The model under review builds one solid part; all positions refer to its coordinate system, in mm. Face numbers are marked on the shaded views. A direction names the side the tool comes from. Round coordinates to 2 decimals unless told otherwise and drop trailing zeros. Loops run counter-clockwise (first coordinate to the right, second up) from the corner with the lowest first, then second, coordinate; pieces in that order, holes last. Notation, with made-up numbers: (4.5, -28) -> (54.5, -28) arc R31 cw to (54.5, 4) -> close; hole circle Ø6 at (-12.75, 68). An arc over 180 degrees is marked (long way). Use CSV: the item, a comma, the result in double quotes. Start each with the question number.
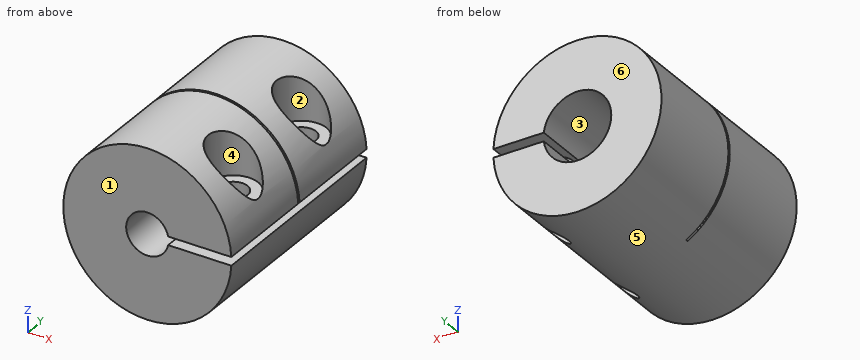
```python
from build123d import *

# Parameters (mm, degrees)
SKETCH1_R                      = 9.925
BOSS_EXTRUDE1_DEPTH            = 12.5
CUT_EXTRUDE5_DEPTH             = 0.125
CUT_EXTRUDE1_REACH             = 30.671
SKETCH3_R                      = 4
SKETCH4_R                      = 2.5
CUT_EXTRUDE2_DEPTH             = 19.878608927
CUT_EXTRUDE6_DEPTH             = 19.795245409
CUT_EXTRUDE6_DEPTH_BACK        = 19.795245409
CBORE_FOR_M3_SHCS1_D           = 3.4
CBORE_FOR_M3_SHCS1_DEPTH       = 9.425
CBORE_FOR_M3_SHCS1_CBORE_D     = 5.9
CBORE_FOR_M3_SHCS1_CBORE_DEPTH = 6
M3X0_5_TAPPED_HOLE1_D          = 2.5


with BuildPart() as part:
    # Sketch1 → Boss-Extrude1 (new, symmetric)
    with BuildSketch(Plane(origin=(0, 0, 0), x_dir=(1, 0, 0), z_dir=(0, 1, 0))):
        with Locations(Location((0, 0, 0), (0, 0, 270))):
            Circle(SKETCH1_R)
    extrude(amount=BOSS_EXTRUDE1_DEPTH, both=True)

    # Sketch10 → Cut-Extrude5 (cut, symmetric)
    with BuildSketch(Plane(origin=(0, 0, 0), x_dir=(1, 0, 0), z_dir=(0, 1, 0))):
        with BuildLine():
            Line((0, -0.5), (0, 0))
            Line((0, 0), (-0.288675135, 0.5))
            Line((-0.288675135, 0.5), (-4.9625, 8.595302133))
            ThreePointArc((-4.9625, 8.595302133), (-5.177499554, -8.467533488), (9.91239754, -0.5))
            Line((9.91239754, -0.5), (0, -0.5))
        make_face()
    extrude(amount=CUT_EXTRUDE5_DEPTH, both=True, mode=Mode.SUBTRACT)

    # Cut-Extrude1: up to this face of the body (flat: up to its plane)
    cut_extrude1_end = Plane(part.part.faces().sort_by_distance((-1.523889636, -0.125, 2.421634097))[0])
    # Sketch3 → Cut-Extrude1 (cut, up to the picked face)
    with BuildSketch(Plane(origin=(0, 12.5, 0), x_dir=(1, 0, 0), z_dir=(0, 1, 0)), mode=Mode.PRIVATE) as cut_extrude1_sk1:
        with Locations(Location((0, 0, 0), (0, 0, 270))):
            Circle(SKETCH3_R)
    cut_extrude1_tool1 = split(extrude(cut_extrude1_sk1.sketch, amount=-CUT_EXTRUDE1_REACH, mode=Mode.PRIVATE), bisect_by=cut_extrude1_end, keep=Keep.BOTH, mode=Mode.PRIVATE)
    add(cut_extrude1_tool1.solids().sort_by(Axis((0, 12.5, 0), (0, -1, 0)))[0], mode=Mode.SUBTRACT)

    # Sketch4 → Cut-Extrude2 (cut, through all)
    with BuildSketch(Plane(origin=(0, -0.125, 0), x_dir=(1, 0, 0), z_dir=(0, 1, 0))):
        with Locations(Location((0, 0, 0), (0, 0, 270))):
            Circle(SKETCH4_R)
    extrude(amount=-CUT_EXTRUDE2_DEPTH, mode=Mode.SUBTRACT)

    # Sketch10<4> → Cut-Extrude6 (cut, two sides: drawn at the far end of the back side and taken through both)
    with BuildSketch(Plane(origin=(0, 0, 0), x_dir=(1, 0, 0), z_dir=(0, 1, 0)).offset(-CUT_EXTRUDE6_DEPTH_BACK)):
        with BuildLine():
            Line((-0.288675135, 0.5), (0, 0))
            Line((0, 0), (0, -0.5))
            Line((0, -0.5), (9.91239754, -0.5))
            ThreePointArc((9.91239754, -0.5), (9.921848885, -0.250079398), (9.925, 0))
            ThreePointArc((9.925, 0), (9.921848885, 0.250079398), (9.91239754, 0.5))
            Line((9.91239754, 0.5), (0, 0.5))
            Line((0, 0.5), (-0.288675135, 0.5))
        make_face()
    extrude(amount=CUT_EXTRUDE6_DEPTH + CUT_EXTRUDE6_DEPTH_BACK, mode=Mode.SUBTRACT)

    # CBORE for M3 SHCS1
    with Locations(Plane.XY.offset(9.925)):
        with Locations((6.180943642, -6.3125), (6.180943642, 6.3125)):
            CounterBoreHole(CBORE_FOR_M3_SHCS1_D / 2, CBORE_FOR_M3_SHCS1_CBORE_D / 2, CBORE_FOR_M3_SHCS1_CBORE_DEPTH, depth=CBORE_FOR_M3_SHCS1_DEPTH)

    # M3x0.5 Tapped Hole1 (through all)
    with Locations(Plane.XY.offset(-0.5)):
        with Locations((6.180943642, 6.3125), (6.180943642, -6.3125)):
            Hole(M3X0_5_TAPPED_HOLE1_D / 2)


solid = part.part
```
1. Take a section at B-B, the plane z = -1.5. Count the separate pieces of the cut face and the enclosed holes in it, then the cut area to 3 significant figures.
2. Take a section at C-C, the plane x = -3. Give the boundary of the cut face in (y, z) (3 decimals).
3. Clearance check with flat-ended pins moving along their axes: P1, Ø4.5, axis at x = 6.18, y = 6.31, coming from the -Z side; P2, Ø6.5, axis at x = 7, y = 7.5, coming from the +Z side; P3, Ø6.5, axis at x = 0, z = 0, coming from the +Y side (3 decimals); P4, Ø10, axis at y = 0.5, z = -1.5, coming from the -X side (3 decimals). State where each tip first meets the part, or that it passes through.
4. For the marked faces 1, 2 and 3, list the 3-axis set-ups (+Z, -Z, +X, -X, +Y, -Y) from which the entire face can be reached by the end or side of a thin tool; tool diameter is ignored.
5. Take a section at A-A, the plane x = 0. Give the boundary of the cut face in (y, z) (3 decimals), then the cut area to 3 significant figures.
6. For line 1 along Z through (x, y) = (0, -10.75) (3 decimals); line 2 along Y through (x, z) = (-6, 2) (3 decimals); line 3 along X through (y, z) = (7.5, 3.5), list the stretches that pass through material, from the lowest coordinate up. Write a range as from..to.
7. The part is to be moulded in two halves that separate along X. For the marked faces 4, 5 and 6, say which applies: pulls with the +X half, pulls with the -X half, needs draft (parallel to the pull), parting line crosses it, or undercut.
Results:
1,separate pieces,"3"
1,enclosed holes,"2"
1,area,"336 mm²"
2,outline,"(-12.5, -9.461) -> (12.5, -9.461) -> (12.5, -2.646) -> (0.125, -2.646) -> (0.125, -5.196) -> (-0.125, -5.196) -> (-0.125, 9.461) -> (-12.5, 9.461) -> close; (0.125, 2.646) -> (12.5, 2.646) -> (12.5, 9.461) -> (0.125, 9.461) -> close"
3,P1,"z = -9.11"
3,P2,"z = 9.17"
3,P3,"y = -0.125"
3,P4,"x = -9.925"
4,face 1,"+Z, -Z, +X, -X, -Y"
4,face 2,"+Z"
4,face 3,"+Y"
5,outline,"(-12.5, -9.925) -> (12.5, -9.925) -> (12.5, -4) -> (-0.125, -4) -> (-0.125, -2.5) -> (-12.5, -2.5) -> close; (-12.5, 2.5) -> (-0.125, 2.5) -> (-0.125, 9.925) -> (-12.5, 9.925) -> close; (0.125, 4) -> (12.5, 4) -> (12.5, 9.925) -> (0.125, 9.925) -> close"
5,area,"332 mm²"
6,line 1,"-9.925..-2.5, 2.5..9.925"
6,line 2,"-12.5..-0.125, 0.125..12.5"
6,line 3,"-9.29..-1.94, 1.94..4.96, 7.4..9.29"
7,face 4,"undercut"
7,face 5,"parting line crosses it"
7,face 6,"needs draft"
